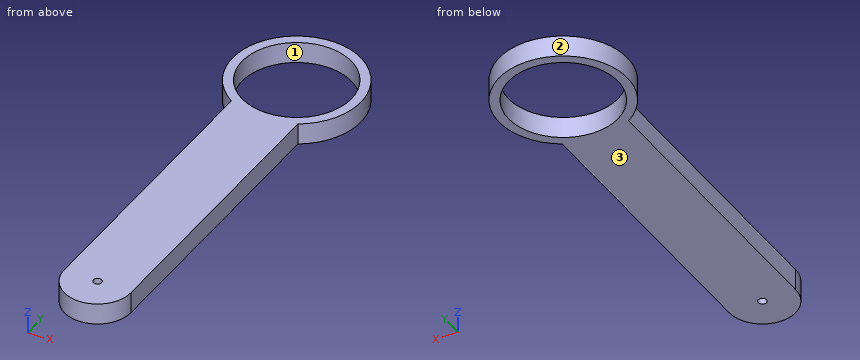
from build123d import *

# Parameters (mm, degrees)
SKETCH_4_R          = 23
EXTRUDE_2_DEPTH     = 9
SKETCH_5_R          = 1.75
CUT_EXTRUDE_1_DEPTH = 10


with BuildPart() as part:
    # 草图4 → 凸台-拉伸2 (new body)
    with BuildSketch(Plane.XY):
        with BuildLine():
            Line((0, 0), (0, 120))
            ThreePointArc((0, 120), (14, 170.086792761), (28, 120))
            Line((28, 120), (28, 0))
            ThreePointArc((28, 0), (14, -14), (0, 0))
        make_face()
        with Locations((14, 143.086792761)):
            Circle(SKETCH_4_R, mode=Mode.SUBTRACT)
    extrude(amount=EXTRUDE_2_DEPTH)

    # 草图5 → 切除-拉伸1 (cut)
    with BuildSketch(Plane(origin=(0, 0, 0), x_dir=(-1, 0, 0), z_dir=(0, 0, -1))):
        with Locations((-14, 0)):
            Circle(SKETCH_5_R)
    extrude(amount=-CUT_EXTRUDE_1_DEPTH, mode=Mode.SUBTRACT)


solid = part.part
The model under review builds one solid part; all positions refer to its coordinate system, in mm. Face numbers are marked on the shaded views. Coordinates: 2 decimals unless noted, no trailing zeros. Write each loop counter-clockwise with the first axis right and the second up, starting at its lowest first coordinate (ties: lowest second). Pieces come first, ordered by that corner, then holes. Notation, with made-up numbers: (84.25, 78.25) -> (133.25, 78.25) arc R6 ccw to (133.25, 85.25) -> close; hole circle Ø2 at (-21.5, -18). An arc over 180 degrees is marked (long way). Answer in a Markdown table with one row per item.
1. Wall thickness on probe 1 along Y at (x, z) = (14, 3); probe 2 along X at (y, z) = (143, 3.5); probe 3 along X at (y, z) = (1.5, 8): over which ranges is each line inside the solid? List them lowest first. Write a range as [from, to].
Answers below:
| item | result |
|---|---|
| probe 1 | y = [-14, -1.75], [1.75, 120.09], [166.09, 170.09] |
| probe 2 | x = [-13, -9], [37, 41] |
| probe 3 | x = [0, 13.1], [14.9, 28] |
2. We need section B-B, the plane x = 2. State the section outline as (y, z) points.
Answers below:
| item | result |
|---|---|
| outline | (-7.21, 0) -> (123.47, 0) -> (123.47, 9) -> (-7.21, 9) -> close; (162.71, 0) -> (167.27, 0) -> (167.27, 9) -> (162.71, 9) -> close |
3. We need section C-C, the plane y = 155. State the section outline as (x, z) points, and give its area (3 significant figures).
Answers below:
| item | result |
|---|---|
| outline | (-10.23, 0) -> (-5.67, 0) -> (-5.67, 9) -> (-10.23, 9) -> close; (33.67, 0) -> (38.23, 0) -> (38.23, 9) -> (33.67, 9) -> close |
| area | 82.0 mm^2 |
4. Draft analysis for pull direction Y (two halves, no side actions). For the marked faces 1, 2 and 3, state which applies: +Y half, -Y half, draft (parallel to the pull), parting line (faces both ways), or undercut.
Answers below:
| item | result |
|---|---|
| face 1 | undercut |
| face 2 | parting line |
| face 3 | draft |
5. We need section D-D, the plane z = 5.25. State the section outline as (x, y) points, and give its area (3 significant figures).
Answers below:
| item | result |
|---|---|
| outline | (0, 0) arc R14 ccw to (28, 0) -> (28, 120) arc R27 ccw (long way) to (0, 120) -> close; hole circle Ø46 at (14, 143.09); hole circle Ø3.5 at (14, 0) |
| area | 4,210 mm^2 |
6. We need section A-A, the plane x = 14. State the section outline as (y, z) points.
Answers below:
| item | result |
|---|---|
| outline | (-14, 0) -> (-1.75, 0) -> (-1.75, 9) -> (-14, 9) -> close; (1.75, 0) -> (120.09, 0) -> (120.09, 9) -> (1.75, 9) -> close; (166.09, 0) -> (170.09, 0) -> (170.09, 9) -> (166.09, 9) -> close |
7. Clearance check with flat-ended pins moving along their axes: pin 1 Ø2.5 at (y, z) = (89.5, 3) entering from +X; pin 2 Ø1 at (x, z) = (0, 2) entering from +Y; pin 3 Ø4 at (x, z) = (-5.5, 5.5) entering from +Y. State where each tip first meets the part, or that it passes through.
Answers below:
| item | result |
|---|---|
| pin 1 | stops at x = 28 |
| pin 2 | stops at y = 166.47 |
| pin 3 | stops at y = 163.65 |
